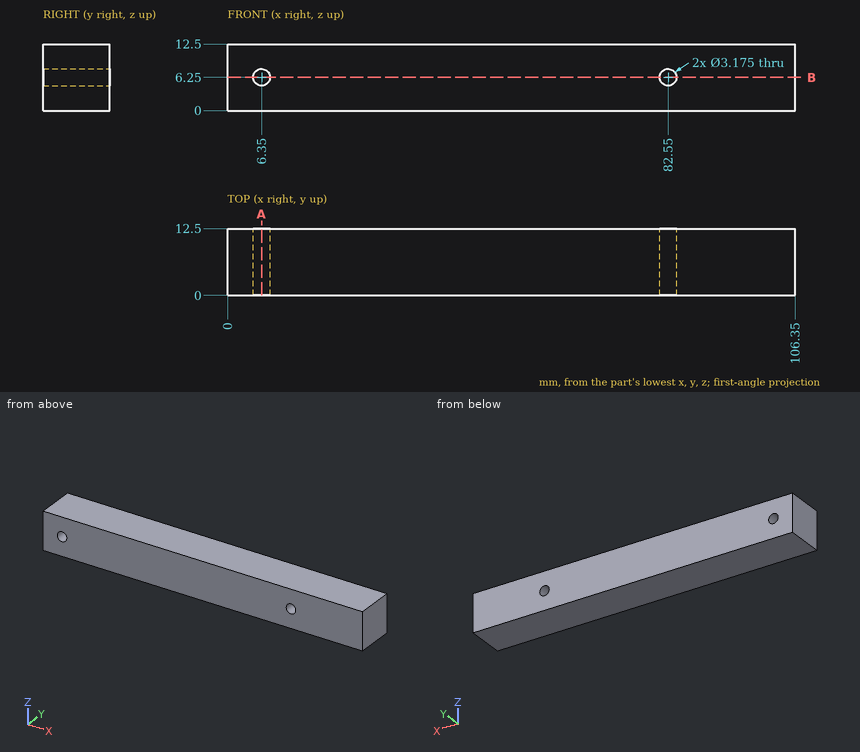
Source: three-view drawing plus pictorial views. Frame: mm from the lowest corner of the part. Round coordinates to 2 decimals unless told otherwise and drop trailing zeros. Loops run counter-clockwise (first coordinate to the right, second up) from the corner with the lowest first, then second, coordinate; pieces in that order, holes last. Notation, with made-up numbers: M -3.5,0.5 L 24.5,0.5 A14 ccw 24.5,21.5 Z; hole C 62,-26.75 d11. An arc over 180 degrees is marked long. Put each result on its own line as item: value. Start each with the question number.
(1) Material intervals for line 1 along Z through (x, y) = (6.35, 7.5); line 2 along X through (y, z) = (4.25, 6.5), sorted ascending. Write a range as [from, to].
(2) Section query B-B (z = 6.25). Return loops of the section in (x, y).
(3) Section query A-A (x = 6.35). Return loops of the section in (y, z), then the cut area to 3 significant figures.
(4) Contact query for a flat-ended pin moving along its axis: pin 1 Ø1.9 at (x, z) = (6.35, 6.25) entering from +Y. Output: stop coordinate, or through.
Findings below:
1. line 1: z = [0, 4.66], [7.84, 12.5]
1. line 2: x = [0, 4.78], [7.92, 80.98], [84.12, 106.35]
2. outline: M 0,0 L 4.76,0 L 4.76,12.5 L 0,12.5 Z; M 7.94,0 L 80.96,0 L 80.96,12.5 L 7.94,12.5 Z; M 84.14,0 L 106.35,0 L 106.35,12.5 L 84.14,12.5 Z
3. outline: M 0,0 L 12.5,0 L 12.5,4.66 L 0,4.66 Z; M 0,7.84 L 12.5,7.84 L 12.5,12.5 L 0,12.5 Z
3. area: 117 mm2
4. pin 1: passes through
